The listing builds one solid part. Answer for the finished solid, in the listing's coordinates (mm). Give positions to 0.01 mm unless a question says otherwise; leave off trailing zeros. Write each loop counter-clockwise with the first axis right and the second up, starting at its lowest first coordinate (ties: lowest second). Pieces come first, ordered by that corner, then holes. Notation, with made-up numbers: (85, -22) -> (116, -22) arc R29 ccw to (116, 15) -> close; hole circle Ø2 at (-26, 68). An arc over 180 degrees is marked (long way). Write each question's results on one line, items separated by ' | '. Start each with the question number.
from build123d import *

# Parameters (mm, degrees)
F1_R     = 0.127
F2_DEPTH = 1.6
F3_R     = 87


with BuildPart() as f2:
    # F1 (on Top) → F2 (new body)
    with BuildSketch(Plane.XY):
        with BuildLine():
            Line((9.9592921435, 26.1), (9.9592921435, 38.446))
            ThreePointArc((9.9592921435, 38.446), (0, 55.696), (-9.9592921435, 38.446))
            Line((-9.9592921435, 38.446), (-9.9592921435, 26.1))
            ThreePointArc((-9.9592921435, 26.1), (-14.6815260775, 8.476383033), (-27.5829091105, -4.425))
            Line((-27.5829091105, -4.425), (-38.2748587457, -10.598))
            ThreePointArc((-38.2748587457, -10.598), (-48.2341508892, -27.848), (-28.3155666021, -27.848))
            Line((-28.3155666021, -27.848), (-17.623616967, -21.675))
            ThreePointArc((-17.623616967, -21.675), (0, -16.952766066), (17.623616967, -21.675))
            Line((17.623616967, -21.675), (28.3155666021, -27.848))
            ThreePointArc((28.3155666021, -27.848), (48.2341508892, -27.848), (38.2748587457, -10.598))
            Line((38.2748587457, -10.598), (27.5829091105, -4.425))
            ThreePointArc((27.5829091105, -4.425), (14.6815260775, 8.476383033), (9.9592921435, 26.1))
        make_face()
        with Locations((-38.2748587457, -22.098)):
            Circle(F1_R, mode=Mode.SUBTRACT)
        with Locations((38.2748587457, -22.098)):
            Circle(F1_R, mode=Mode.SUBTRACT)
        with Locations((0, 44.196)):
            Circle(F1_R, mode=Mode.SUBTRACT)
    extrude(amount=F2_DEPTH)

    # F3
    f3_edges = [f2.edges().sort_by_distance(p)[0] for p in [
        (-28.315567, -27.848, 0.8),
        (-38.274859, -10.598, 0.8),
        (28.315567, -27.848, 0.8),
        (38.274859, -10.598, 0.8),
        (9.959292, 38.446, 0.8),
        (-9.959292, 38.446, 0.8),
    ]]
    fillet(f3_edges, radius=F3_R)


solid = f2.part
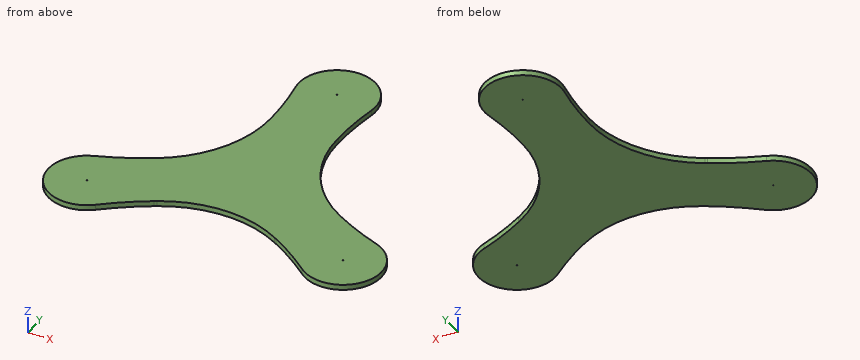
1. Section C-C (y = -0.5) is taken. Write down the section's boundary in (x, z), then the cut area to 3 significant figures.
2. Each of these flat-tipped pins is pushed along its axis until it touches: pin 1 Ø0.8 at (y, z) = (26.5, 1) entering from -X; pin 2 Ø6 at (x, y) = (16, 45) entering from +Z. Where does it stop, or does it pass through?
3. Section A-A (z = 0.3) is taken. Write down the section's boundary in (x, y) (3 decimals).
4. Consider probe 1 along Y at (x, z) = (0, 0.7); probe 2 along X at (y, z) = (-27.5, 1.45); probe 3 along X at (y, z) = (-7, 0.4). Determine where each line is inside the solid, lowest interval first. Write a range as [from, to].
5. Section B-B (x = -2) is taken. Write down the section's boundary in (y, z), then the cut area to 3 significant figures.
Results:
1) outline: (-22.08, 0) -> (22.08, 0) -> (22.08, 1.6) -> (-22.08, 1.6) -> close | area: 70.7 mm²
2) pin 1: stops at x = -9.96 | pin 2: passes through
3) outline: (-42.18, -11.281) arc R11.5 ccw (long way) to (-30.86, -30.888) arc R87 cw to (-18.267, -22.046) -> (-17.624, -21.675) arc R35.247 cw to (17.624, -21.675) -> (18.267, -22.046) arc R87 cw to (30.86, -30.888) arc R11.5 ccw (long way) to (42.18, -11.281) arc R87 cw to (28.226, -4.796) -> (27.583, -4.425) arc R35.247 cw to (9.959, 26.1) -> (9.959, 26.842) arc R87 cw to (11.32, 42.17) arc R11.5 ccw (long way) to (-11.32, 42.17) arc R87 cw to (-9.959, 26.842) -> (-9.959, 26.1) arc R35.247 cw to (-27.583, -4.425) -> (-28.226, -4.796) arc R87 cw to start; hole circle Ø0.254 at (-38.275, -22.098); hole circle Ø0.254 at (0, 44.196); hole circle Ø0.254 at (38.275, -22.098)
4) probe 1: y = [-16.95, 44.07], [44.32, 55.7] | probe 2: x = [-48.43, -26.58], [26.58, 48.43] | probe 3: x = [-32.29, 32.29]
5) outline: (-17.01, 0) -> (55.52, 0) -> (55.52, 1.6) -> (-17.01, 1.6) -> close | area: 116 mm²
